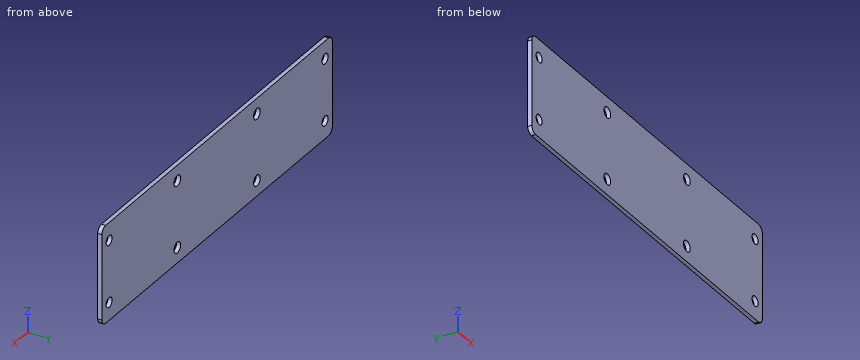
```python
from build123d import *

# Parameters (mm, degrees)
SKETCH2_W           = 121.6
SKETCH2_H           = 31.5
SKETCH2_R           = 1.6
BOSS_EXTRUDE1_DEPTH = 1.35
FILLET1_R           = 2
SKETCH3_R           = 1.75
CUT_EXTRUDE1_DEPTH  = 63.821373751


with BuildPart() as part:
    # Sketch2 → Boss-Extrude1 (new body)
    with BuildSketch(Plane(origin=(0, 0, 0), x_dir=(1, 0, 0), z_dir=(0, 1, 0))):
        Rectangle(SKETCH2_W, SKETCH2_H)
        with Locations(Location((-57, 10, 0), (0, 0, 270))):
            Circle(SKETCH2_R, mode=Mode.SUBTRACT)
        with Locations(Location((-57, -10, 0), (0, 0, 270))):
            Circle(SKETCH2_R, mode=Mode.SUBTRACT)
        with Locations(Location((57, 10, 0), (0, 0, 270))):
            Circle(SKETCH2_R, mode=Mode.SUBTRACT)
        with Locations(Location((57, -10, 0), (0, 0, 270))):
            Circle(SKETCH2_R, mode=Mode.SUBTRACT)
    extrude(amount=-BOSS_EXTRUDE1_DEPTH)

    # Fillet1
    fillet1_edges = [part.edges().sort_by_distance(p)[0] for p in [
        (-60.8, -0.675, -15.75),
        (60.8, -0.675, -15.75),
        (60.8, -0.675, 15.75),
        (-60.8, -0.675, 15.75),
    ]]
    fillet(fillet1_edges, radius=FILLET1_R)

    # Sketch3 → Cut-Extrude1 (cut, through all)
    with BuildSketch(Plane(origin=(0, 0, 0), x_dir=(1, 0, 0), z_dir=(0, 1, 0))):
        with Locations(Location((-21, -10.75, 0), (0, 0, 270))):
            Circle(SKETCH3_R)
        with Locations(Location((21, -10.75, 0), (0, 0, 270))):
            Circle(SKETCH3_R)
        with Locations(Location((21, 10.75, 0), (0, 0, 270))):
            Circle(SKETCH3_R)
        with Locations(Location((-21, 10.75, 0), (0, 0, 270))):
            Circle(SKETCH3_R)
    extrude(amount=-CUT_EXTRUDE1_DEPTH, mode=Mode.SUBTRACT)


solid = part.part
```
Could you check a few things on this model? Use its own coordinates, in mm. Coordinates: 2 decimals unless noted, no trailing zeros. Write each loop counter-clockwise with the first axis right and the second up, starting at its lowest first coordinate (ties: lowest second). Pieces come first, ordered by that corner, then holes. Notation, with made-up numbers: (40.25, 74) - (51.25, 74) arc R26 ccw to (51.25, 113) - close; hole circle Ø3 at (20.5, 21). An arc over 180 degrees is marked (long way). Use a Markdown table: item, result.
Q1. Please list where these lines run through material, in increasing order: L1, parallel to X at y = -0.65, z = 11; L2, parallel to X at y = -0.2, z = 12; L3, parallel to X at y = -0.45, z = -10.75.
Geometry check:
| item | result |
|---|---|
| L1 | x = -60.8 to -58.25, -55.75 to -22.73, -19.27 to 19.27, 22.73 to 55.75, 58.25 to 60.8 |
| L2 | x = -60.8 to -22.22, -19.78 to 19.78, 22.22 to 60.8 |
| L3 | x = -60.8 to -58.41, -55.59 to -22.75, -19.25 to 19.25, 22.75 to 55.59, 58.41 to 60.8 |
Q2. I'm going to push a flat-ended pin straight in: pin 1 Ø5.5 at (x, z) = (21, -10.75) entering from +Y. Where does the tip first touch, or does it pass through?
Geometry check:
| item | result |
|---|---|
| pin 1 | stops at y = 0 |
Q3. Imagine slicing it at A-A (x = 21). List the corners of the cut face in (y, z) for me.
Geometry check:
| item | result |
|---|---|
| outline | (-1.35, -15.75) - (0, -15.75) - (0, -12.5) - (-1.35, -12.5) - close; (-1.35, -9) - (0, -9) - (0, 9) - (-1.35, 9) - close; (-1.35, 12.5) - (0, 12.5) - (0, 15.75) - (-1.35, 15.75) - close |
